from build123d import *

# Parameters (mm, degrees)
EXTRUDE_1_DEPTH     = 5.5
SKETCH_4_R          = 1
SKETCH_4_W          = 5.5
SKETCH_4_H          = 5.5
CUT_EXTRUDE_2_DEPTH = 129.993216876
FILLET_1_R          = 5
FILLET_2_R          = 5
SKETCH_5_R          = 0.75
CUT_EXTRUDE_3_DEPTH = 129.993216876
SKETCH_6_R          = 1.05
CUT_EXTRUDE_4_DEPTH = 129.993216876
SKETCH_7_W          = 15
SKETCH_7_H          = 90
CUT_EXTRUDE_5_DEPTH = 129.993216876
SKETCH_8_W          = 29.991103618
SKETCH_8_H          = 3
CUT_EXTRUDE_6_DEPTH = 129.993216876
SKETCH_9_R          = 1.05
SKETCH_9_W          = 12.2
SKETCH_9_H          = 22.5
CUT_EXTRUDE_7_DEPTH = 129.993216876
FILLET_3_R          = 5
SKETCH_10_R         = 1.05
CUT_EXTRUDE_8_DEPTH = 129.993216876


with BuildPart() as part:
    # ｽｹｯﾁ1 → ﾎﾞｽ - 押し出し1 (new body)
    with BuildSketch(Plane.XY):
        with BuildLine():
            Line((31, 120), (-47, 120))
            Line((-47, 120), (-47, 65))
            Line((-47, 65), (-19, 53.216373532))
            Line((-19, 53.216373532), (-19, 23.216373532))
            ThreePointArc((-19, 23.216373532), (0, -30), (19, 23.216373532))
            Line((19, 23.216373532), (19, 57.75))
            Line((19, 57.75), (31, 67.75))
            Line((31, 67.75), (31, 120))
        make_face()
    extrude(amount=EXTRUDE_1_DEPTH)

    # ｽｹｯﾁ4 → ｶｯﾄ - 押し出し2 (cut, through all)
    with BuildSketch(Plane.XY.offset(5.5)):
        with Locations((14, 63)):
            Circle(SKETCH_4_R)
        with Locations((14, 83)):
            Circle(SKETCH_4_R)
        with Locations((14, 73)):
            Circle(SKETCH_4_R)
        with Locations(Location((-14, 83, 0), (0, 0, 180))):
            Circle(SKETCH_4_R)
        with Locations(Location((-14, 73, 0), (0, 0, 180))):
            Circle(SKETCH_4_R)
        with Locations(Location((-14, 63, 0), (0, 0, 180))):
            Circle(SKETCH_4_R)
        with Locations((22.75, 112)):
            Rectangle(SKETCH_4_W, SKETCH_4_H)
        with Locations((22.75, 73)):
            Rectangle(SKETCH_4_W, SKETCH_4_H)
    extrude(amount=-CUT_EXTRUDE_2_DEPTH, mode=Mode.SUBTRACT)

    # ﾌｨﾚｯﾄ1
    fillet_1_edges = [part.edges().sort_by_distance(p)[0] for p in [
        (-47, 65, 2.75),
    ]]
    fillet(fillet_1_edges, radius=FILLET_1_R)

    # ﾌｨﾚｯﾄ2
    fillet_2_edges = [part.edges().sort_by_distance(p)[0] for p in [
        (-19, 53.216373532, 2.75),
    ]]
    fillet(fillet_2_edges, radius=FILLET_2_R)

    # ｽｹｯﾁ5 → ｶｯﾄ - 押し出し3 (cut, through all)
    with BuildSketch(Plane.XY.offset(5.5)):
        with Locations((14.45, 0)):
            Circle(SKETCH_5_R)
        with Locations((-14.45, 0)):
            Circle(SKETCH_5_R)
    extrude(amount=-CUT_EXTRUDE_3_DEPTH, mode=Mode.SUBTRACT)

    # ｽｹｯﾁ6 → ｶｯﾄ - 押し出し4 (cut, through all)
    with BuildSketch(Plane.XY.offset(5.5)):
        with Locations((-24.425038206, -12.880897043)):
            Circle(SKETCH_6_R)
        with Locations((-21.701843031, -17.074249883)):
            Circle(SKETCH_6_R)
        with Locations(Location((24.425038206, -12.880897043, 0), (0, 0, 180))):
            Circle(SKETCH_6_R)
        with Locations(Location((21.701843031, -17.074249883, 0), (0, 0, 180))):
            Circle(SKETCH_6_R)
    extrude(amount=-CUT_EXTRUDE_4_DEPTH, mode=Mode.SUBTRACT)

    # ｽｹｯﾁ7 → ｶｯﾄ - 押し出し5 (cut, through all)
    with BuildSketch(Plane.XY.offset(5.5)):
        with Locations((0, 68)):
            Rectangle(SKETCH_7_W, SKETCH_7_H)
    extrude(amount=-CUT_EXTRUDE_5_DEPTH, mode=Mode.SUBTRACT)

    # ｽｹｯﾁ8 → ｶｯﾄ - 押し出し6 (cut, through all)
    with BuildSketch(Plane.XY.offset(5.5)):
        with Locations((-33.995551809, 75)):
            Rectangle(SKETCH_8_W, SKETCH_8_H)
    extrude(amount=-CUT_EXTRUDE_6_DEPTH, mode=Mode.SUBTRACT)

    # ｽｹｯﾁ9 → ｶｯﾄ - 押し出し7 (cut, through all)
    with BuildSketch(Plane.XY.offset(5.5)):
        with Locations((-36.5, 66.3)):
            Circle(SKETCH_9_R)
        with Locations((-36.5, 94)):
            Circle(SKETCH_9_R)
        with Locations((-36.5, 80.15)):
            Rectangle(SKETCH_9_W, SKETCH_9_H)
    extrude(amount=-CUT_EXTRUDE_7_DEPTH, mode=Mode.SUBTRACT)

    # ﾌｨﾚｯﾄ3
    fillet_3_edges = [part.edges().sort_by_distance(p)[0] for p in [
        (31, 67.75, 2.75),
    ]]
    fillet(fillet_3_edges, radius=FILLET_3_R)

    # ｽｹｯﾁ10 → ｶｯﾄ - 押し出し8 (cut, through all)
    with BuildSketch(Plane.XY.offset(5.5)):
        with Locations((16, 22)):
            Circle(SKETCH_10_R)
        with Locations((16, 26)):
            Circle(SKETCH_10_R)
        with Locations((16, 30)):
            Circle(SKETCH_10_R)
        with Locations((16, 34)):
            Circle(SKETCH_10_R)
        with Locations((16, 38)):
            Circle(SKETCH_10_R)
        with Locations((16, 42)):
            Circle(SKETCH_10_R)
        with Locations((16, 46)):
            Circle(SKETCH_10_R)
        with Locations((16, 50)):
            Circle(SKETCH_10_R)
        with Locations(Location((-16, 50, 0), (0, 0, 180))):
            Circle(SKETCH_10_R)
        with Locations(Location((-16, 46, 0), (0, 0, 180))):
            Circle(SKETCH_10_R)
        with Locations(Location((-16, 42, 0), (0, 0, 180))):
            Circle(SKETCH_10_R)
        with Locations(Location((-16, 38, 0), (0, 0, 180))):
            Circle(SKETCH_10_R)
        with Locations(Location((-16, 34, 0), (0, 0, 180))):
            Circle(SKETCH_10_R)
        with Locations(Location((-16, 30, 0), (0, 0, 180))):
            Circle(SKETCH_10_R)
        with Locations(Location((-16, 26, 0), (0, 0, 180))):
            Circle(SKETCH_10_R)
        with Locations(Location((-16, 22, 0), (0, 0, 180))):
            Circle(SKETCH_10_R)
        with Locations((16, 54)):
            Circle(SKETCH_10_R)
        with Locations(Location((-16, 54, 0), (0, 0, 180))):
            Circle(SKETCH_10_R)
    extrude(amount=-CUT_EXTRUDE_8_DEPTH, mode=Mode.SUBTRACT)


solid = part.part
Source: CAD feature listing. Evaluate the final solid. Frame: model axes, mm. A direction names the side the tool comes from. Round coordinates to 2 decimals unless told otherwise and drop trailing zeros. Loops run counter-clockwise (first coordinate to the right, second up) from the corner with the lowest first, then second, coordinate; pieces in that order, holes last. Notation, with made-up numbers: (-11, -13.5) -> (31, -13.5) arc R22 ccw to (31, 5.5) -> close; hole circle Ø11 at (74.5, -33). An arc over 180 degrees is marked (long way). Answer as a JSON object with one key per item and string values. Group by question number.
Q1. Section query C-C (z = 1). State how many separate pieces and enclosed holes the cut face has, plus the area to 3 significant figures.
Q2. Access query for faces 1 (the flat face through (-45, 76.5, 3)), 2 (the flat face through (-42.6, 71, 3)), 3 (the flat face through (-9, 46, 5.5)). Directions: +Z, -Z, +X, -X, +Y, -Y. A direction counts if a zero-diameter tool reaches every point of the face in a straight line with its end or side. Return the directions, or none.
Q3. Section query A-A (y = 97). Output: boundary loops of the cut face in (x, z).
Q4. Mould query, pull axis X, two halves, no side actions, for faces 4 (the cylindrical face through (-19.86, 52.7, 2.79)), 5 (the flat face through (25.5, 112, 3)), 6 (the flat face through (19, 40, 3)), 7 (the flat face through (-30.4, 84, 3)). Classes: pulls with the +X half, pulls with the -X half, needs draft (parallel to the pull), parting line crosses it, or undercut.
Q5. Section query B-B (x = 0). Output: boundary loops of the cut face in (y, z), plus the area to 3 significant figures.
Q6. Ray query, line 1 (X direction, y = 73, z = 2.5); line 2 (X direction, y = 83, z = 2.65); line 3 (X direction, y = 88, z = 1.85). Return the intervals inside material, ascending. Write a range as from..to.
Q7. Contact query for flat-ended pins moving along their axis: P1, Ø3, axis at y = 55, z = 1.5, coming from the -X side; P2, Ø1.5, axis at y = 65, z = 3, coming from the +X side; P3, Ø2.5, axis at x = 16, y = 54, coming from the +Z side; P4, Ø2, axis at x = -28, z = 2.5, coming from the -Y side. Output: stop coordinate, or through.
Completed:
{
 "1": {"separate pieces": "1", "enclosed holes": "35", "area": "6,880 mm²"},
 "2": {"face 1": "+Z, -Z, -X", "face 2": "+Z, -Z", "face 3": "+Z, +X, -X, +Y, -Y"},
 "3": {"outline": "(-47, 0) -> (-7.5, 0) -> (-7.5, 5.5) -> (-47, 5.5) -> close; (7.5, 0) -> (31, 0) -> (31, 5.5) -> (7.5, 5.5) -> close"},
 "4": {"face 4": "pulls with the -X half", "face 5": "undercut", "face 6": "pulls with the +X half", "face 7": "undercut"},
 "5": {"outline": "(-30, 0) -> (23, 0) -> (23, 5.5) -> (-30, 5.5) -> close; (113, 0) -> (120, 0) -> (120, 5.5) -> (113, 5.5) -> close", "area": "330 mm²"},
 "6": {"line 1": "-47..-42.6, -30.4..-15, -13..-7.5, 7.5..13, 15..20, 25.5..31", "line 2": "-47..-42.6, -30.4..-15, -13..-7.5, 7.5..13, 15..31", "line 3": "-47..-42.6, -30.4..-7.5, 7.5..31"},
 "7": {"P1": "x = -26.8", "P2": "x = 28.6", "P3": "z = 5.5", "P4": "y = -13.08"}
}
